Here's how the part is built. I have some questions about the finished solid (model axes, mm). Face numbers are marked on the shaded views. A direction names the side the tool comes from. Give positions to 0.01 mm unless a question says otherwise; leave off trailing zeros. Loops run counter-clockwise (first coordinate to the right, second up) from the corner with the lowest first, then second, coordinate; pieces in that order, holes last. Notation, with made-up numbers: M 5,22 L 25,22 A20 cw 25,60 Z; hole C 84.5,13.25 d6. An arc over 180 degrees is marked long. Write item = value, one per line. Start each with the question number.
```python
from build123d import *

# Parameters (mm, degrees)
BOSS_EXTRUDE1_DEPTH   = 127
BOSS_EXTRUDE1_2_DEPTH = 127
BOSS_EXTRUDE7_DEPTH   = 127
BOSS_EXTRUDE7_2_DEPTH = 127
SKETCH10_W            = 685.8
SKETCH10_H            = 685.8
BOSS_EXTRUDE8_DEPTH   = 76.2
SKETCH11_W            = 482.6
SKETCH11_H            = 596.9
CUT_EXTRUDE3_DEPTH    = 50.8
BOSS_EXTRUDE9_DEPTH   = 635
BOSS_EXTRUDE11_DEPTH  = 101.6
BOSS_EXTRUDE12_DEPTH  = 101.6
CUT_EXTRUDE4_DEPTH    = 1531.798988842


with BuildPart() as part:
    # Sketch1 → Boss-Extrude1 (new body)
    with BuildSketch(Plane(origin=(0, 0, 0), x_dir=(0, 0, -1), z_dir=(1, 0, 0))):
        Polygon((0, 0), (228.6, 0), (228.6, 127), (127, 127), (127, 431.8), (330.2, 431.8), (330.2, 558.8), (0, 558.8), align=None)
    extrude(amount=BOSS_EXTRUDE1_DEPTH)



with BuildPart() as body_2:
    # Sketch1 → Boss-Extrude1 2 (new body)
    with BuildSketch(Plane(origin=(0, 0, 0), x_dir=(0, 0, -1), z_dir=(1, 0, 0))):
        Polygon((635, 558.8), (635, 0), (304.8, 0), (304.8, 127), (508, 127), (508, 431.8), (406.4, 431.8), (406.4, 558.8), align=None)
    extrude(amount=BOSS_EXTRUDE1_2_DEPTH)


with BuildPart() as body_3:
    # Sketch9 → Boss-Extrude7 (new body)
    with BuildSketch(Plane(origin=(635, 0, 0), x_dir=(0, 0, -1), z_dir=(1, 0, 0))):
        Polygon((127, 431.8), (330.2, 431.8), (330.2, 558.8), (0, 558.8), (0, 0), (228.6, 0), (228.6, 127), (127, 127), align=None)
    extrude(amount=-BOSS_EXTRUDE7_DEPTH)


with BuildPart() as body_4:
    # Sketch9 → Boss-Extrude7 2 (new body)
    with BuildSketch(Plane(origin=(635, 0, 0), x_dir=(0, 0, -1), z_dir=(1, 0, 0))):
        Polygon((406.4, 558.8), (406.4, 431.8), (508, 431.8), (508, 127), (304.8, 127), (304.8, 0), (635, 0), (635, 558.8), align=None)
    extrude(amount=-BOSS_EXTRUDE7_2_DEPTH)


with BuildPart() as part_1:
    add(part.part)

    add(body_2.part)  # Boss-Extrude8 merges body 2

    add(body_3.part)  # Boss-Extrude8 merges body 3

    add(body_4.part)  # Boss-Extrude8 merges body 4
    # Sketch10 → Boss-Extrude8 (add)
    with BuildSketch(Plane(origin=(0, 558.8, 0), x_dir=(1, 0, 0), z_dir=(0, 1, 0))):
        with Locations((317.5, 317.5)):
            Rectangle(SKETCH10_W, SKETCH10_H)
    extrude(amount=BOSS_EXTRUDE8_DEPTH)

    # Sketch11 → Cut-Extrude3 (cut)
    with BuildSketch(Plane(origin=(0, 635, 0), x_dir=(1, 0, 0), z_dir=(0, 1, 0))):
        with Locations((317.5, 273.05)):
            Rectangle(SKETCH11_W, SKETCH11_H)
    extrude(amount=-CUT_EXTRUDE3_DEPTH, mode=Mode.SUBTRACT)

    # Sketch13 → Boss-Extrude9 (add)
    with BuildSketch(Plane(origin=(635, 0, 0), x_dir=(0, 0, -1), z_dir=(1, 0, 0))):
        Polygon((660.4, 635), (742.98211211, 1219.2), (692.18211211, 1219.2), (571.5, 635), align=None)
    extrude(amount=-BOSS_EXTRUDE9_DEPTH)

    # Sketch15 → Boss-Extrude11 (add)
    with BuildSketch(Plane(origin=(660.4, 0, 0), x_dir=(0, 0, -1), z_dir=(1, 0, 0))):
        Polygon((-25.4, 635), (-25.4, 889), (457.2, 889), (457.2, 812.8), (50.8, 812.8), (50.8, 635), align=None)
    extrude(amount=-BOSS_EXTRUDE11_DEPTH)

    # Sketch16 → Boss-Extrude12 (add)
    with BuildSketch(Plane(origin=(-25.4, 0, 0), x_dir=(0, 0, -1), z_dir=(1, 0, 0))):
        Polygon((50.8, 635), (50.8, 812.8), (457.2, 812.8), (457.2, 889), (-25.4, 889), (-25.4, 635), align=None)
    extrude(amount=BOSS_EXTRUDE12_DEPTH)

    # Sketch17 → Cut-Extrude4 (cut, through all)
    with BuildSketch(Plane(origin=(0, -87.23785604, -422.302482176), x_dir=(1, 0, 0), z_dir=(0, 0.20230522100715992, 0.9793225196804392))):
        Polygon((90.072307692, 1168.922071162), (153.572307692, 1168.922071162), (237.392307692, 970.802071162), (285.75, 1085.102071162), (349.25, 1085.102071162), (390.546160735, 970.802071162), (474.366160735, 1168.922071162), (537.866160735, 1168.922071162), (409.066806467, 864.487233803), (345.566806467, 864.487233803), (307.466806467, 1016.440282577), (269.366806467, 864.487233803), (205.866806467, 864.487233803), align=None)
    extrude(amount=-CUT_EXTRUDE4_DEPTH, mode=Mode.SUBTRACT)


solid = part_1.part
```
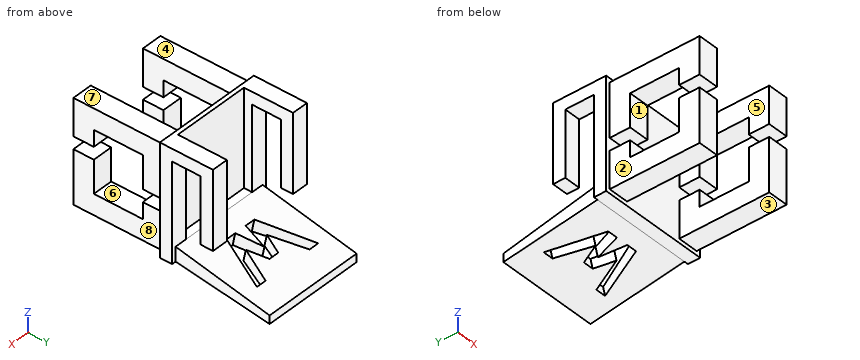
Q1. If I drill on line 1 along Y through (x, z) = (44.5, -330); line 2 along X through (y, z) = (415, -603); line 3 along Z through (x, y) = (108.5, 358.5), over which ranges is the centre line in solid material (lowest first)?
Q2. If we section it at A-A, the plane y = 175: List the corners of the cut face in (x, z) for me, then the cut area to 3 significant figures.
Q3. If we section it at C-C, the plane x = 222: List the corners of the cut face in (y, z) for me, then the cut area to 3 significant figures.
Q4. Will these pins go through, and if not, where does the flat tip stop? pin 1 (1.5 mm diameter, centred on x = 277, y = 1051.5, fed in from +Z); pin 2 (1.5 mm diameter, centred on x = 389.5, y = 972, fed in from +Z); pin 3 (1 mm diameter, centred on x = 557, y = 1052.5, fed in from -Z).
Q5. On a 3-axis mill with a long thin cutter (end or side, diameter ignored), from which of +Z, -Z, +X, -X, +Y, -Y can I reach the whole of each face in a straight line? I mean the marked faces 1, 2, 3, 4 and 5. Say none if no direction works.
Q6. If we section it at B-B, the plane z = -164.5: State how many separate pieces and enclosed holes the cut face has, then the cut area to 3 significant figures.
Q7. We'd pull the mould along Z, two halves only. Please class the marked faces 6, 7 and 8: pulls with the +Z half, pulls with the -Z half, needs draft (parallel to the pull), parting line crosses it, or undercut.
Q8. If we section it at D-D, the plane z = -273: List the corners of the cut face in (x, y) for me.
Resolved:
q1.line_1 = 0 to 127, 431.8 to 635, 812.8 to 889
q1.line_2 = 0 to 127, 508 to 635
q1.line_3 = -635 to -508, -127 to 0
q2.outline = M 0,-635 L 127,-635 L 127,-508 L 0,-508 Z; M 0,-127 L 127,-127 L 127,0 L 0,0 Z; M 508,-635 L 635,-635 L 635,-508 L 508,-508 Z; M 508,-127 L 635,-127 L 635,0 L 508,0 Z
q2.area = 64,500 mm²
q3.outline = M 558.8,-660.4 L 635,-660.4 L 743.16,-675.69 L 759.37,-597.19 L 635,-571.5 L 584.2,-571.5 L 584.2,25.4 L 558.8,25.4 Z; M 884.73,-695.7 L 1219.2,-742.98 L 1219.2,-692.18 L 899.12,-626.06 Z
q3.area = 51,900 mm²
q4.pin_1 = -657.38
q4.pin_2 = -640.96
q4.pin_3 = -719.49
q5.face_1 = +X, -X
q5.face_2 = +Z, -Z, -X, -Y
q5.face_3 = -Z, +X, -X, -Y
q5.face_4 = +Z, +X, -X, -Y
q5.face_5 = +Z, -Z, -Y
q6.separate_pieces = 5
q6.enclosed_holes = 0
q6.area = 108,000 mm²
q7.face_6 = undercut
q7.face_7 = pulls with the +Z half
q7.face_8 = needs draft
q8.outline = M -25.4,558.8 L 0,558.8 L 0,431.8 L 127,431.8 L 127,558.8 L 508,558.8 L 508,431.8 L 635,431.8 L 635,558.8 L 660.4,558.8 L 660.4,635 L 558.8,635 L 558.8,584.2 L 76.2,584.2 L 76.2,635 L -25.4,635 Z; M -25.4,812.8 L 76.2,812.8 L 76.2,889 L -25.4,889 Z; M 558.8,812.8 L 660.4,812.8 L 660.4,889 L 558.8,889 Z
